Here's the drawing with two shaded views (mm, measured from the low corner). I have some questions. A direction names the side the tool comes from. Round coordinates to 2 decimals unless told otherwise and drop trailing zeros. Order: outer loops, then holes, each group sorted by start corner. A loop starts at its lowest first (then second) coordinate and runs counter-clockwise, first axis right, second up. Notation, with made-up numbers: (73, 24.5) -> (81, 24.5) arc R30 ccw to (81, 51.5) -> close; hole circle Ø5 at (38.25, -5.5). An arc over 180 degrees is marked (long way). Use a Markdown table: item, result. Add a question column.
Q1. I need wall thicknesses on line 1 along Y through (x, z) = (14.5, 1.4); line 2 along Y through (x, z) = (32.7, 0.9); line 3 along X through (y, z) = (13, 3.75). Which ranges of each line are inside material? Lowest first, please. Write a range as [from, to].
Q2. If we section it at C-C on y = 13.5: List the corners of the cut face in (x, z) for me, plus the area to 3 significant figures.
Q3. If we section it at A-A on y = 23.75: List the corners of the cut face in (x, z) for me, plus the area to 3 significant figures.
Q4. I'm going to push flat-ended pins straight in: pin 1 Ø2 at (y, z) = (7.5, 6) entering from +X; pin 2 Ø5 at (x, y) = (32.7, 23.75) entering from +Z; pin 3 Ø5 at (x, y) = (20.5, 5) entering from +Z (1 decimal). Where does each tip first touch, or does it pass through?
Q5. If we section it at D-D on z = 6.2: List the corners of the cut face in (x, y) for me, plus the area to 3 significant figures.
Q6. For the marked faces 1, 2, 3 and 4, which set-ups out of +Z, -Z, +X, -X, +Y, -Y let a thin tool reach every point of the face, with its end or its side?
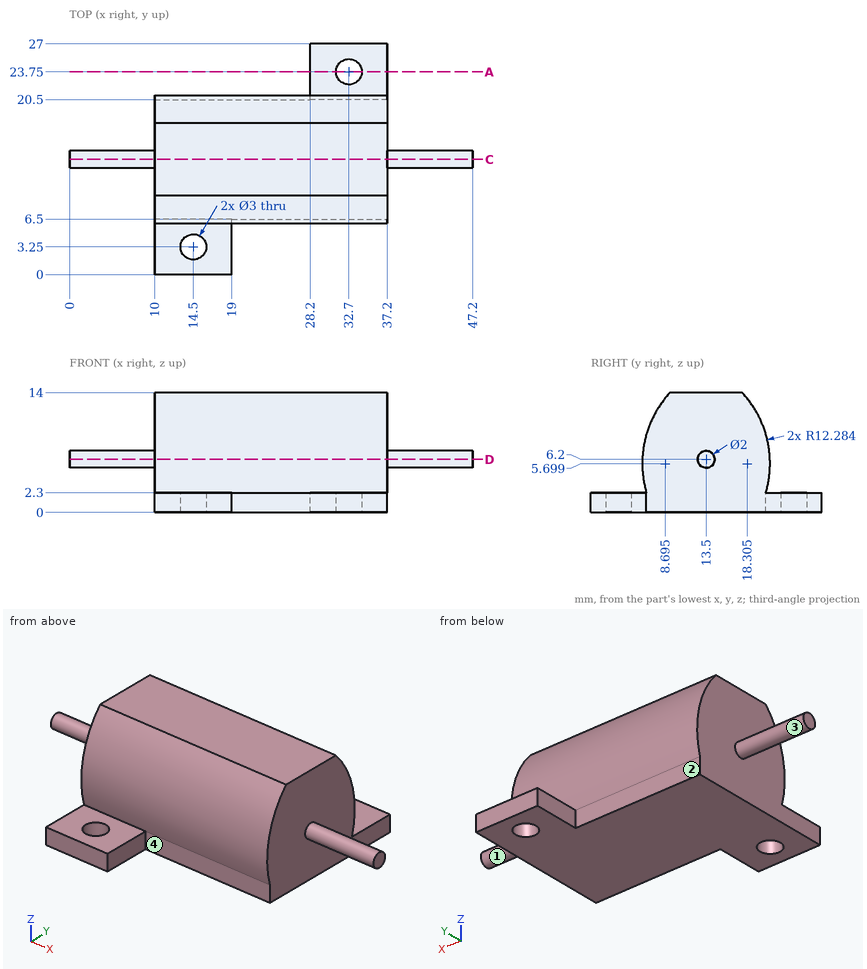
Answer below:
| question | item | result |
|---|---|---|
| 1 | line 1 | [0, 1.75], [4.75, 20.5] |
| 1 | line 2 | [6.5, 22.25], [25.25, 27] |
| 1 | line 3 | [10, 37.2] |
| 2 | outline | (0, 5.2) -> (10, 5.2) -> (10, 0) -> (37.2, 0) -> (37.2, 5.2) -> (47.2, 5.2) -> (47.2, 7.2) -> (37.2, 7.2) -> (37.2, 14) -> (10, 14) -> (10, 7.2) -> (0, 7.2) -> close |
| 2 | area | 421 mm² |
| 3 | outline | (28.2, 0) -> (31.2, 0) -> (31.2, 2.3) -> (28.2, 2.3) -> close; (34.2, 0) -> (37.2, 0) -> (37.2, 2.3) -> (34.2, 2.3) -> close |
| 3 | area | 13.8 mm² |
| 4 | pin 1 | x = 37.2 |
| 4 | pin 2 | z = 2.3 |
| 4 | pin 3 | z = 11.5 |
| 5 | outline | (0, 12.5) -> (10, 12.5) -> (10, 6.03) -> (37.2, 6.03) -> (37.2, 12.5) -> (47.2, 12.5) -> (47.2, 14.5) -> (37.2, 14.5) -> (37.2, 20.97) -> (10, 20.97) -> (10, 14.5) -> (0, 14.5) -> close |
| 5 | area | 446 mm² |
| 6 | face 1 | +X |
| 6 | face 2 | -Z, -X, +Y |
| 6 | face 3 | -X |
| 6 | face 4 | -Z, +X, -Y |
